```python
from build123d import *

# Parameters (mm, degrees)
SKETCH1_R           = 27.686
BOSS_EXTRUDE1_DEPTH = 12.319
SKETCH2_W           = 9.906
SKETCH2_H           = 15.113
SKETCH3_R           = 3.175
CUT_EXTRUDE1_DEPTH  = 25.638


with BuildPart() as part:
    # Sketch1 → Boss-Extrude1 (new body, symmetric)
    with BuildSketch(Plane.XY):
        Circle(SKETCH1_R)
    extrude(amount=BOSS_EXTRUDE1_DEPTH, both=True)

    # Sketch2 → Cut-Revolve1 (revolve, cut)
    with BuildSketch(Plane(origin=(0, 0, 0), x_dir=(0, 0, -1), z_dir=(1, 0, 0))):
        with Locations((-7.366, 15.9385)):
            Rectangle(SKETCH2_W, SKETCH2_H)
    cut_revolve1 = revolve(axis=Axis((0, 0, 0), (0, 0, 1)), mode=Mode.SUBTRACT)

    # Sketch3 → Cut-Extrude1 (cut, through all)
    with BuildSketch(Plane.XY.offset(12.319)):
        Circle(SKETCH3_R)
    extrude(amount=-CUT_EXTRUDE1_DEPTH, mode=Mode.SUBTRACT)

    # Mirror1: Cut-Revolve1 across plane
    add(cut_revolve1.mirror(Plane.XY), mode=Mode.SUBTRACT)


solid = part.part
```
Source: CAD feature listing. Evaluate the final solid. Frame: model axes, mm. A direction names the side the tool comes from. Round coordinates to 2 decimals unless told otherwise and drop trailing zeros. Write each loop counter-clockwise with the first axis right and the second up, starting at its lowest first coordinate (ties: lowest second). Pieces come first, ordered by that corner, then holes. Notation, with made-up numbers: M 78,48.25 L 85,48.25 A19 cw 85,66.25 Z; hole C 42,60.5 d8. An arc over 180 degrees is marked long. Answer as a JSON object with one key per item and string values. Group by question number.
(1) Mould query, pull axis Y, two halves, no side actions, for faces 1 (the cylindrical face through (-0.69, -3.1, 0.17)), 2 (the cylindrical face through (14.884, 23.345, 0.172)), 3 (the flat face through (0, -4, 12.319)), 4 (the cylindrical face through (14.3, -18.64, 7.3)). Classes: +Y half, -Y half, draft (parallel to the pull), parting line (faces both ways), or undercut.
(2) Section query D-D on x = -18.5. Output: boundary loops of the cut face in (y, z).
(3) Section query C-C on z = -5.25. Output: boundary loops of the cut face in (x, y) (3 decimals).
(4) First-contact query: pin 1 (8 mm diameter, centred on x = 5, z = -2.5, fed in from +Y); pin 2 (4 mm diameter, centred on x = 0, y = 0, fed in from +Z); pin 3 (1 mm diameter, centred on y = -1, z = -6.5, fed in from +X); pin 4 (4 mm diameter, centred on x = 17.5, y = 0.5, fed in from -Z). Flat tips, straight axial feed; report the tip coordinate or a pass-through.
(5) Reachability of faces 5 (the flat face through (10, 0, -2.413)), 6 (the cylindrical face through (-2.5, 8, 7.3)), 7 (the flat face through (-12.4, -20.4, -12.319)) from +Z, -Z, +X, -X, +Y, -Y: full face, straight path, thin tool, end or side. Return the list, or none.
(6) Ray query, line 1 (Y direction, x = 0, z = 9.25) (3 decimals); line 2 (Z direction, x = 16.5, y = 14); line 3 (X direction, y = -4, z = 9.5). Return the intervals inside material, ascending. Write a range as [from, to].
(7) Section query A-A on x = 0. Output: boundary loops of the cut face in (y, z) (3 decimals), then the cut area to 3 significant figures.
Computed values:
{
 "1": {"face 1": "undercut", "face 2": "parting line", "face 3": "draft", "face 4": "undercut"},
 "2": {"outline": "M -20.6,-12.32 L -14.48,-12.32 L -14.48,-2.41 L 14.48,-2.41 L 14.48,-12.32 L 20.6,-12.32 L 20.6,12.32 L 14.48,12.32 L 14.48,2.41 L -14.48,2.41 L -14.48,12.32 L -20.6,12.32 Z"},
 "3": {"outline": "C 0,0 d55.372; C 0,0 d16.764; hole C 0,0 d46.99; hole C 0,0 d6.35"},
 "4": {"pin 1": "y = 27.67", "pin 2": "through", "pin 3": "x = 27.68", "pin 4": "z = -2.41"},
 "5": {"face 5": "-Z", "face 6": "+Z", "face 7": "-Z, +X, -X, +Y, -Y"},
 "6": {"line 1": "[-27.686, -23.495], [-8.382, -3.175], [3.175, 8.382], [23.495, 27.686]", "line 2": "[-2.41, 2.41]", "line 3": "[-27.4, -23.15], [-7.37, 7.37], [23.15, 27.4]"},
 "7": {"outline": "M -27.686,-12.319 L -23.495,-12.319 L -23.495,-2.413 L -8.382,-2.413 L -8.382,-12.319 L -3.175,-12.319 L -3.175,12.319 L -8.382,12.319 L -8.382,2.413 L -23.495,2.413 L -23.495,12.319 L -27.686,12.319 Z; M 3.175,-12.319 L 8.382,-12.319 L 8.382,-2.413 L 23.495,-2.413 L 23.495,-12.319 L 27.686,-12.319 L 27.686,12.319 L 23.495,12.319 L 23.495,2.413 L 8.382,2.413 L 8.382,12.319 L 3.175,12.319 Z", "area": "609 mm^2"}
}
